from build123d import *

# Parameters (mm, degrees)
F0_R     = 44.5
F0_R_2   = 2.25
F1_DEPTH = 2
F2_R     = 35.5
F3_DEPTH = 22
F3_TAPER = 22
F4_R     = 33.5
F4_R_2   = 26.6114230316
F5_DEPTH = 32


with BuildPart() as f1:
    # F0 (on Top) → F1 (new body)
    with BuildSketch(Plane.XY):
        Circle(F0_R)
        with Locations((0, -41.25)):
            Circle(F0_R_2, mode=Mode.SUBTRACT)
        with Locations((-41.25, 0)):
            Circle(F0_R_2, mode=Mode.SUBTRACT)
        with Locations((41.25, 0)):
            Circle(F0_R_2, mode=Mode.SUBTRACT)
        with Locations((0, 41.25)):
            Circle(F0_R_2, mode=Mode.SUBTRACT)
    extrude(amount=F1_DEPTH)

    # F2 (on face) → F3 (join)
    with BuildSketch(Plane(origin=(0, 0, 0), x_dir=(1, 0, 0), z_dir=(0, 0, -1))):
        Circle(F2_R)
    extrude(amount=F3_DEPTH, taper=F3_TAPER)

    # F4 (on face) → F5 (join)
    with BuildSketch(Plane(origin=(0, 0, -22), x_dir=(1, 0, 0), z_dir=(0, 0, -1))):
        Circle(F4_R)
        Circle(F4_R_2, mode=Mode.SUBTRACT)
        Circle(F4_R_2)
    extrude(amount=F5_DEPTH)

    # F6 (on Front) → F7 (revolve, cut)
    with BuildSketch(Plane.XZ):
        with BuildLine():
            Line((0, 0), (0, -6.9301972061))
            ThreePointArc((0, -6.9301972061), (3.2915026221, -7.638694584), (6, -9.638694584))
            ThreePointArc((6, -9.638694584), (18.6340040872, -6.3979944791), (30, 0))
            Line((30, 0), (30, 3))
            Line((30, 3), (0, 3))
            Line((0, 3), (0, 0))
        make_face()
    revolve(axis=Axis((0, 0, -5), (0, 0, -1)), mode=Mode.SUBTRACT)


solid = f1.part
The model under review builds one solid part; all positions refer to its coordinate system, in mm. A direction names the side the tool comes from. Coordinates: 2 decimals unless noted, no trailing zeros. Loops run counter-clockwise (first coordinate to the right, second up) from the corner with the lowest first, then second, coordinate; pieces in that order, holes last. Notation, with made-up numbers: (17.25, 85.25) -> (73.25, 85.25) arc R21 ccw to (73.25, 97.25) -> close; hole circle Ø2 at (-16.5, -3). An arc over 180 degrees is marked (long way). Use a Markdown table: item, result. Add a question column.
1. Clearance check with flat-ended pins moving along their axes: pin 1 Ø5 at (x, y) = (0, 41.25) entering from -Z; pin 2 Ø2.5 at (x, y) = (-41.25, 0) entering from -Z; pin 3 Ø8 at (x, z) = (8.5, -5.5) entering from -Y; pin 4 Ø20 at (x, y) = (-9, 16.5) entering from +Z. State where each tip first meets the part, or that it passes through.
2. Add section A-A on x = -41.25. Write out the cut boundary in (y, z), plus the area to 3 significant figures.
3. Add section B-B on x = 0. Write out the cut boundary in (y, z).
4. Machinability: for faces 4 (the face through (-29.97, -1.32, 1.01)), 5 (the face through (0, -39, 1)), 6 (the face through (25.794, -8.123, -20.932)), which of the approach directions +Z, -Z, +X, -X, +Y, -Y give a long, thin tool a straight path to every point of the face, cutting with its end or side? Answer none if there is none.
5. Add section D-D on z = -3.5. Write out the cut boundary in (x, y).
6. Draft analysis for pull direction X (two halves, no side actions). For faces 1 (the face through (-13.4, 33.2, 0)), 2 (the face through (-0.29, 43.48, 0.99)), 3 (the face through (-7.262, 32.703, -37.776)), state which applies: pulls with the +X half, pulls with the -X half, needs draft (parallel to the pull), parting line crosses it, or undercut.
7. To check wall thickness, follow line 1 (Y direction, x = 0, z = 1); line 2 (Z direction, x = -4, y = 36.5); line 3 (Z direction, x = -22, y = 21.5). State the ranges of each line that lie inside material, in increasing order.
Returned:
| question | item | result |
|---|---|---|
| 1 | pin 1 | stops at z = 0 |
| 1 | pin 2 | passes through |
| 1 | pin 3 | stops at y = -34.07 |
| 1 | pin 4 | stops at z = -0.88 |
| 2 | outline | (-16.69, 0) -> (-2.25, 0) -> (-2.25, 2) -> (-16.69, 2) -> close; (2.25, 0) -> (16.69, 0) -> (16.69, 2) -> (2.25, 2) -> close |
| 2 | area | 57.8 mm² |
| 3 | outline | (-44.5, 0) -> (-43.5, 0) -> (-43.5, 2) -> (-44.5, 2) -> close; (-39, 0) -> (-35.5, 0) -> (-26.61, -22) -> (-33.5, -22) -> (-33.5, -54) -> (33.5, -54) -> (33.5, -22) -> (26.61, -22) -> (35.5, 0) -> (39, 0) -> (39, 2) -> (30, 2) -> (30, 0) arc R50 cw to (6, -9.64) arc R8 ccw to (-6, -9.64) arc R50 cw to (-30, 0) -> (-30, 2) -> (-39, 2) -> close; (43.5, 0) -> (44.5, 0) -> (44.5, 2) -> (43.5, 2) -> close |
| 4 | face 4 | +Z |
| 4 | face 5 | +Z, -Z |
| 4 | face 6 | none |
| 5 | outline | circle Ø68.17 at (0, 0); hole circle Ø49.31 at (0, 0) |
| 6 | face 1 | needs draft |
| 6 | face 2 | undercut |
| 6 | face 3 | parting line crosses it |
| 7 | line 1 | y = -44.5 to -43.5, -39 to -30, 30 to 39, 43.5 to 44.5 |
| 7 | line 2 | z = 0 to 2 |
| 7 | line 3 | z = -54 to -22, -11.73 to 2 |
